Geometry check sheet. Reference: the model listing, model coordinates, mm. Coordinates: 2 decimals unless noted, no trailing zeros. Write each loop counter-clockwise with the first axis right and the second up, starting at its lowest first coordinate (ties: lowest second). Pieces come first, ordered by that corner, then holes.
from build123d import *

# Parameters (mm, degrees)
SKETCH1_W           = 9.84142284
SKETCH1_H           = 9.84142284
BOSS_EXTRUDE1_DEPTH = 15
CUT_EXTRUDE1_DEPTH  = 0.3


with BuildPart() as part:
    # Sketch1 → Boss-Extrude1 (new body)
    with BuildSketch(Plane(origin=(0, 0, 0), x_dir=(1, 0, 0), z_dir=(0, 1, 0))):
        Rectangle(SKETCH1_W, SKETCH1_H)
        with BuildLine():
            Line((-1.865475811, 2.509444822), (1.865475811, 2.509444822))
            ThreePointArc((1.865475811, 2.509444822), (0, -3.290555178), (-1.865475811, 2.509444822))
        make_face(mode=Mode.SUBTRACT)
    extrude(amount=BOSS_EXTRUDE1_DEPTH)

    # Sketch2 → Cut-Extrude1 (cut)
    with BuildSketch(Plane.XY.offset(4.92071142)):
        Polygon((-1.296362428, 9.754838654), (0.677996546, 9.754838654), (0.677996546, 9.395864295), (-0.982259864, 9.395864295), (-0.982259864, 8.318941219), (0.677996546, 8.318941219), (0.677996546, 7.95996686), (-0.982259864, 7.95996686), (-0.982259864, 6.613813013), (0.677996546, 6.613813013), (0.677996546, 6.254838654), (-1.296362428, 6.254838654), align=None)
    extrude(amount=-CUT_EXTRUDE1_DEPTH, mode=Mode.SUBTRACT)


solid = part.part
1. Draft check along Z on faces 1 (the cylindrical face through (0.11, 7.4, 3.29)), 2 (the flat face through (0, 7, -4.921)), 3 (the flat face through (0, 0, -3)), 4 (the flat face through (0, 7, -2.509)). Enter one of: released by +Z, released by -Z, zero draft, split by the parting line, or undercut.
Computed values:
face 1: undercut
face 2: released by -Z
face 3: zero draft
face 4: undercut
2. Sectioned sample at A-A, the plane x = -3. Record the boundary of the cut face in (y, z).
Computed values:
outline: (0, -4.92) - (15, -4.92) - (15, -1.02) - (0, -1.02) - close; (0, 1.2) - (15, 1.2) - (15, 4.92) - (0, 4.92) - close
3. Sectioned sample at C-C, the plane y = 9. Record the boundary of the cut face in (x, z), and give its area (3 significant figures).
Computed values:
outline: (-4.92, -4.92) - (4.92, -4.92) - (4.92, 4.92) - (-0.98, 4.92) - (-0.98, 4.62) - (-1.3, 4.62) - (-1.3, 4.92) - (-4.92, 4.92) - close; hole (-1.87, -2.51) - (1.87, -2.51) arc R3.2 ccw (long way) to start
area: 66.1 mm2
4. Thickness scan on line 1 along Z through (x, y) = (0, 7.5); line 2 along Z through (x, y) = (-1.5, 1.25); line 3 along X through (y, z) = (10.75, 1.5). Record the ranges inside material, lowest first.
Computed values:
line 1: z = -4.92 to -2.51, 3.29 to 4.92
line 2: z = -4.92 to -2.51, 2.92 to 4.92
line 3: x = -4.92 to -2.87, 2.87 to 4.92
5. Sectioned sample at D-D, the plane x = 0. Record the boundary of the cut face in (y, z).
Computed values:
outline: (0, -4.92) - (15, -4.92) - (15, -2.51) - (0, -2.51) - close; (0, 3.29) - (15, 3.29) - (15, 4.92) - (9.75, 4.92) - (9.75, 4.62) - (9.4, 4.62) - (9.4, 4.92) - (8.32, 4.92) - (8.32, 4.62) - (7.96, 4.62) - (7.96, 4.92) - (6.61, 4.92) - (6.61, 4.62) - (6.25, 4.62) - (6.25, 4.92) - (0, 4.92) - close
6. Sectioned sample at B-B, the plane z = 0.25. Record the boundary of the cut face in (x, y).
Computed values:
outline: (-4.92, 0) - (-3.2, 0) - (-3.2, 15) - (-4.92, 15) - close; (3.2, 0) - (4.92, 0) - (4.92, 15) - (3.2, 15) - close
